Solid Edge part; units mm, degrees
sketch "Sketch1" plane through (-10.5, 25.05, 4.8) normal (0, 0, 1) x (0, 1, 0)
  line L0 (-19.8, 27.5) -> (30.8492, -9.504)
  line L1 (-35.05, 27.5) -> (-19.8, 27.5)
  line L2 (-35.05, -22.5) -> (-35.05, 27.5)
  line L3 (-22.8, -22.5) -> (-35.05, -22.5)
  arc A0 (-22.8, -22.5) -> (-19.8, -22.5) centre (-21.3, -22.5) cw
  line L4 (-19.8, -22.5) -> (-19.8, -27.5)
  line L5 (-19.8, -27.5) -> (-10, -27.5)
  line L6 (-10, -27.5) -> (-10, -22.5)
  arc A1 (-10, -22.5) -> (-7, -22.5) centre (-8.5, -22.5) cw
  line L7 (-7, -22.5) -> (22.15, -22.5)
  arc A2 (22.15, -22.5) -> (25.15, -22.5) centre (23.65, -22.5) cw
  line L8 (25.15, -27.5) -> (25.15, -22.5)
  line L9 (34.95, -27.5) -> (25.15, -27.5)
  line L10 (34.95, -22.5) -> (34.95, -27.5)
  line L11 (34.95, -17.5786) -> (34.95, -22.5)
  arc A3 (30.8492, -9.504) -> (34.95, -17.5786) centre (24.95, -17.5786) cw
extrude "ExtrudedProtrusion_3" add sketch "Sketch1" against normal blind 5
sketch "Sketch2" plane through (-13, 0, 2.3) normal (0, 0, 1) x (0, 1, 0)
  circle A0 centre (0.15, 8) radius 1.55
extrude "ExtrudedCutout_14" cut sketch "Sketch2" against normal blind 5
fillet "Round_3" radius 3 1 edges at (-38, -10, 2.3)
sketch "Sketch3" plane through (-10.5, 25, -0.2) normal (0, 0, -1) x (-1, 0, 0)
  arc A0 (-19.4524, 9.225) -> (-18, 10.35) centre (-18, 8.85) cw
  line L0 (-18, 10.35) -> (-16.5, 10.35)
  arc A1 (-16.5, 10.35) -> (-15.048, 9.2266) centre (-16.5, 8.85) cw
  arc A2 (-16.5, 4.9) -> (-15.048, 6.0234) centre (-16.5, 6.4) ccw
  line L1 (-18, 4.9) -> (-16.5, 4.9)
  arc A3 (-19.4524, 6.025) -> (-18, 4.9) centre (-18, 6.4) ccw
  line L2 (-22.5, 6.025) -> (-19.4524, 6.025)
  line L3 (-22.5, 7.625) -> (-22.5, 6.025)
  line L4 (-22.5, 7.625) -> (-22.5, 9.225)
  line L5 (-22.5, 9.225) -> (-19.4524, 9.225)
  arc A4 (-15.048, 9.2265) -> (-15.048, 6.0235) centre (-15.0254, 7.625) cw
extrude "Cutout1" cut sketch "Sketch3" against normal blind 5
sketch "Sketch4" plane through (-10.5, 25, 4.8) normal (0, 0, 1) x (0.5899241, 0.8074587, 0)
  line L0 (-2.674, -29.8188) -> (-32.1702, 10.5541)
  line L1 (-32.1702, 10.5541) -> (-40.4063, 4.5369)
  line L2 (-40.4063, 4.5369) -> (-10.9101, -35.836)
  line L3 (-10.9101, -35.836) -> (-2.674, -29.8188)
extrude "ExtrudedCutout_16" cut sketch "Sketch4" against normal blind 2.5
hole "Hole_4" at (-21, 0.15, -0.2) direction (0, 0, 1) diameter 3.2 end up to next countersink diameter 6.94 countersink angle 90
properties material "Polycarbonate"
The listing builds one solid part. Answer for the finished solid, in the listing's coordinates (mm). A direction names the side the tool comes from. Give positions to 0.01 mm unless a question says otherwise; leave off trailing zeros. Write each loop counter-clockwise with the first axis right and the second up, starting at its lowest first coordinate (ties: lowest second). Pieces come first, ordered by that corner, then holes. Notation, with made-up numbers: (61.25, 77) -> (65.25, 77) arc R12 cw to (65.25, 83) -> close; hole circle Ø7 at (43, 22). An arc over 180 degrees is marked (long way). Use a Markdown table: item, result.
(1) For faces 1 (the flat face through (7, 35.35, 2)), 2 (the flat face through (12, 24, 2)), 3 (the flat face through (-13, 0, 2.3)), determine the directions among +Z, -Z, +X, -X, +Y, -Y from which every point of the face is accessible in a straight line to the end or side of a thin tool.
Return value:
| item | result |
|---|---|
| face 1 | +Z, -Z |
| face 2 | +Z, -Z, +X |
| face 3 | +Z, +X, -X |
(2) Section C-C, the plane y = 24 is taken. Determine the outline of the cut face in (x, z), then the cut area to 3 significant figures.
Return value:
| item | result |
|---|---|
| outline | (-24.3, -0.2) -> (12, -0.2) -> (12, 4.8) -> (-24.3, 4.8) -> close |
| area | 182 mm2 |
(3) Section B-B, the plane y = 6.5 is taken. Determine the outline of the cut face in (x, z), then the cut area to 3 significant figures.
Return value:
| item | result |
|---|---|
| outline | (-37.09, -0.2) -> (17, -0.2) -> (17, 4.8) -> (-37.09, 4.8) -> close |
| area | 270 mm2 |
(4) Determine the mould class of faces 4 (the flat face through (12, -5, 2)), 5 (the flat face through (12, 60, 2)), 6 (the cylindrical face through (-19.414, -0.058, 1.981)) for opening direction Y: released by +Y, released by -Y, zero draft, split by the parting line, or undercut.
Return value:
| item | result |
|---|---|
| face 4 | zero draft |
| face 5 | released by +Y |
| face 6 | undercut |
(5) Flat-ended cylindrical pins translate along their axes: P1, Ø1.2, axis at x = -19.5, z = 3, coming from the +Y side; P2, Ø2.5, axis at x = 15, z = 1.5, coming from the -Y side; P3, Ø3.5, axis at x = -21, y = 0.15, coming from the +Z side. Find the tip coordinate at first contact, or state that the pin passes through.
Return value:
| item | result |
|---|---|
| P1 | y = 31.39 |
| P2 | y = 5.25 |
| P3 | z = 2.3 |
(6) Find the intervals of material crossed by probe 1 along X at (y, z) = (0.15, 1.95); probe 2 along Y at (x, z) = (12.5, 3.5); probe 3 along Z at (x, y) = (-5.5, 0.5), in increasing order. Write a range as from..to.
Return value:
| item | result |
|---|---|
| probe 1 | -38..-22.6, -19.4..12 |
| probe 2 | 5.25..15.05, 50.2..60 |
| probe 3 | -0.2..2.3 |
(7) Section A-A, the plane x = -21 is taken. Determine the outline of the cut face in (y, z).
Return value:
| item | result |
|---|---|
| outline | (-10, -0.2) -> (-3.32, -0.2) -> (-1.45, 1.67) -> (-1.45, 2.3) -> (-4.95, 2.3) -> (-4.95, 4.8) -> (-10, 4.8) -> close; (1.75, 1.67) -> (3.62, -0.2) -> (28.52, -0.2) -> (28.52, 4.8) -> (5.25, 4.8) -> (5.25, 2.3) -> (1.75, 2.3) -> close |
